The figure shows three views and two pictorial views of one solid part (mm, origin at its lowest corner). Answer the questions. A direction names the side the tool comes from. Coordinates: 2 decimals unless noted, no trailing zeros. Order: outer loops, then holes, each group sorted by start corner. A loop starts at its lowest first (then second) coordinate and runs counter-clockwise, first axis right, second up.
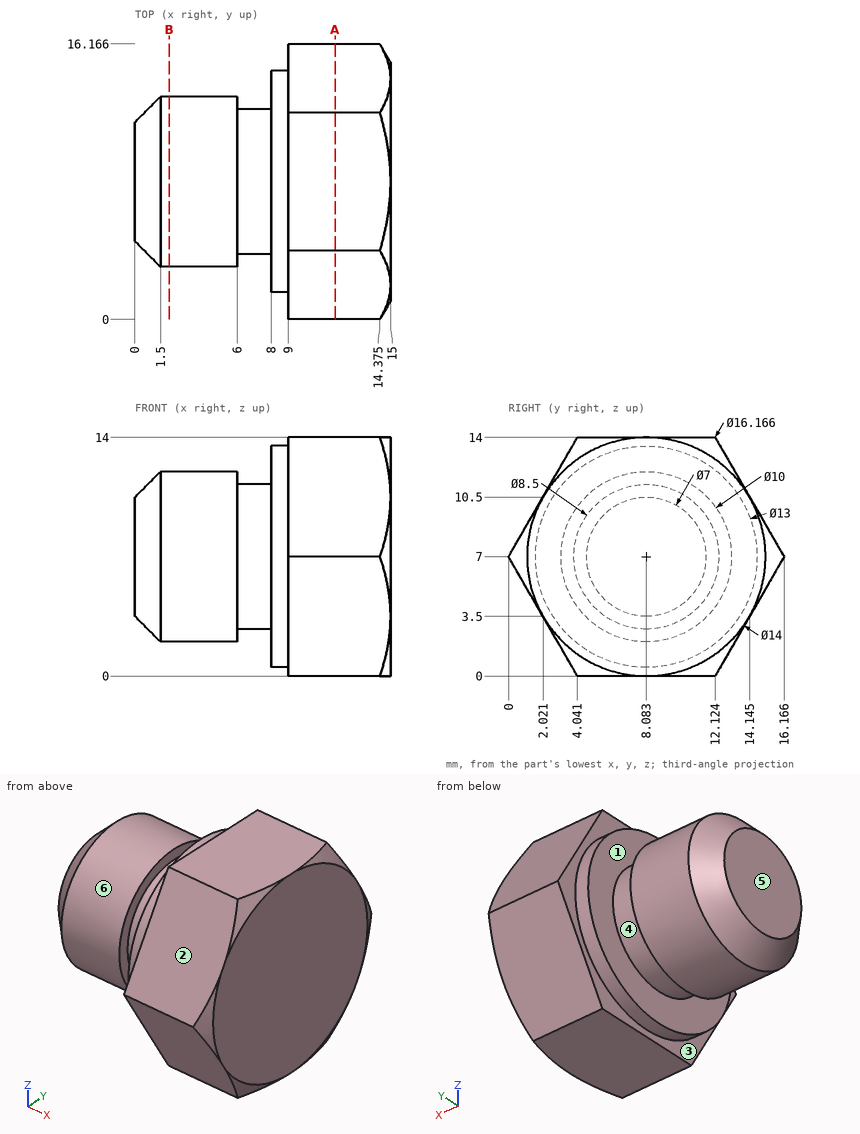
Q1. The part is cut by section A-A, the plane x = 11.75. Determine the outline of the cut face in (y, z) (1 decimal), then the cut area to 3 significant figures.
Q2. The part is cut by section B-B, the plane x = 2. Determine the outline of the cut face in (y, z).
Q3. Which of the six approach directions +Z, -Z, +X, -X, +Y, -Y give full straight-line access (tool end or side, diameter ignored) to the marked faces 1, 2 and 3?
Q4. Determine the mould class of the marked faces 4, 5 and 6 for opening direction X: +X half, -X half, draft (parallel to the pull), parting line (faces both ways), or undercut.
Q5. Straight lines are drawn through the part: L1, parallel to Z at x = 12.5, y = 3.75 (1 decimal); L2, parallel to X at y = 14.25, z = 9.75; L3, parallel to X at y = 10.25, z = 9.75. For each, find the intervals that lie inside material, in ascending order.
Q6. Each of these flat-tipped pins is pushed along its axis until it touches: P1, Ø2, axis at x = 12, y = 14, coming from the -Z side (1 decimal); P2, Ø2, axis at x = 11, z = 12, coming from the -Y side; P3, Ø5, axis at x = 4, y = 3.5, coming from the -Z side (1 decimal). Where does it stop, or does it pass through?
Computed values:
1. outline: (0, 7) - (4, 0) - (12.1, 0) - (16.2, 7) - (12.1, 14) - (4, 14) - close
1. area: 170 mm2
2. outline: circle Ø10 at (8.08, 7)
3. face 1: none
3. face 2: +Z, +X, -X, -Y
3. face 3: -X
4. face 4: undercut
4. face 5: -X half
4. face 6: draft
5. L1: z = 0.5 to 13.5
5. L2: x = 9 to 15
5. L3: x = 0 to 15
6. P1: stops at z = 1.5
6. P2: stops at y = 2.31
6. P3: stops at z = 2.5
